from build123d import *

# Parameters (mm, degrees)
F3_DEPTH     = 3.5
F4_SIZE      = 1
F5_SIZE      = 0.5
F6_T4_DEPTH  = 8.4221557451
F6_T11_DEPTH = 13.7150489639
F6_T21_DEPTH = 8.4221557451
F6_T28_DEPTH = 8.4221557451
F6_T35_DEPTH = 13.7150489639
F6_T45_DEPTH = 8.4221557451
F7_R         = 1.5
F8_R         = 1
F9_DEPTH     = 25


# Not quite as in the source:
# - a fillet or chamfer that OpenCascade refuses, or shapes differently, is made with other operations: its cross-section is extruded or revolved along the edge and cut away or added


with BuildPart() as f1:
    # F0 (on Front) → F1 (revolve)
    with BuildSketch(Plane.XZ):
        Polygon((0, 7), (0, 0), (5.5, 0), (5.5, 3.5), (6.5, 3.5), (6.5, 7), align=None)
    revolve(axis=Axis((0, 0, 5.0261294236), (0, 0, 1)))

    # F2 (on Front) → F3 (join, symmetric)
    with BuildSketch(Plane.XZ):
        Polygon((3.5, 0), (-3.5, 0), (-3.5, -2.5), (-2, -2.5), (-2, -7.5), (-3.5, -7.5), (-3.5, -9.5), (3.5, -9.5), (3.5, -7.5), (2, -7.5), (2, -2.5), (3.5, -2.5), align=None)
    extrude(amount=F3_DEPTH, both=True)

    # F4
    f4_edges = [f1.edges().sort_by_distance(p)[0] for p in [
        (3.5, -3.5, -1.25),
        (3.5, 3.5, -1.25),
        (-3.5, 3.5, -1.25),
        (-3.5, -3.5, -1.25),
        (-3.5, -3.5, -8.5),
        (3.5, -3.5, -8.5),
        (-3.5, 3.5, -8.5),
        (3.5, 3.5, -8.5),
    ]]
    chamfer(f4_edges, length=F4_SIZE)

    # F5
    f5_edges = [f1.edges().sort_by_distance(p)[0] for p in [
        (2, -3.5, -5),
        (-2, -3.5, -5),
        (-2, 3.5, -5),
        (2, 3.5, -5),
    ]]
    chamfer(f5_edges, length=F5_SIZE)

    # F6: chamfer of 1.5 on 6 edges, made by hand


with BuildPart() as f6_tool2:
    # F6_s3 → F6_t4 (new body)
    with BuildSketch(Plane(origin=(3.7276817198, -3.7276817198, 0), x_dir=(0, 0, 1), z_dir=(-0.7071067812, 0.7071067812, 0))):
        Polygon((-7.5, -5.0355339059), (-6, -3.5355339059), (-7.5, -3.5355339059), align=None)
    extrude(amount=F6_T4_DEPTH)

    split(bisect_by=Plane.XZ.offset(3.5), keep=Keep.BOTTOM)

    split(bisect_by=Plane(origin=(-3, -3, 0), x_dir=(0, 0, 1), z_dir=(0.7071067812, 0.7071067812, 0)), keep=Keep.TOP)

    split(bisect_by=Plane(origin=(2, 0, -2), x_dir=(0, 1, 0), z_dir=(0.7071067812, 0, -0.7071067812)), keep=Keep.TOP)


with BuildPart() as f1_1:
    add(f1.part)

    # F6_t1: union F6_tool2
    add(f6_tool2.part)


with BuildPart() as f6_tool9:
    # F6_s10 → F6_t11 (new body)
    with BuildSketch(Plane.XZ.offset(-6.8575244819)):
        Polygon((-3.5, -7.5), (-2, -6), (-2, -7.5), align=None)
    extrude(amount=F6_T11_DEPTH)

    split(bisect_by=Plane.XZ.offset(3.5), keep=Keep.BOTTOM)

    split(bisect_by=Plane(origin=(-3, -3, 0), x_dir=(0, 0, 1), z_dir=(0.7071067812, 0.7071067812, 0)), keep=Keep.TOP)

    split(bisect_by=Plane.XZ.offset(-3.5), keep=Keep.TOP)

    split(bisect_by=Plane(origin=(-3, 3, 0), x_dir=(0, 0, 1), z_dir=(0.7071067812, -0.7071067812, 0)), keep=Keep.TOP)

    split(bisect_by=Plane(origin=(0.8713203436, -0.8713203436, -1.232233047), x_dir=(0.7071067812, 0.7071067812, 0), z_dir=(0.5, -0.5, -0.7071067812)), keep=Keep.TOP)

    split(bisect_by=Plane(origin=(0.8713203436, 0.8713203436, -1.232233047), x_dir=(-0.7071067812, 0.7071067812, 0), z_dir=(0.5, 0.5, -0.7071067812)), keep=Keep.TOP)


with BuildPart() as f1_2:
    add(f1_1.part)

    # F6_t8: union F6_tool9
    add(f6_tool9.part)


with BuildPart() as f6_tool19:
    # F6_s20 → F6_t21 (new body)
    with BuildSketch(Plane(origin=(3.7276817198, 3.7276817198, 0), x_dir=(0, 0, 1), z_dir=(-0.7071067812, -0.7071067812, 0))):
        Polygon((-7.5, 5.0355339059), (-6, 3.5355339059), (-7.5, 3.5355339059), align=None)
    extrude(amount=F6_T21_DEPTH)

    split(bisect_by=Plane.XZ.offset(-3.5), keep=Keep.TOP)

    split(bisect_by=Plane(origin=(-3, 3, 0), x_dir=(0, 0, 1), z_dir=(0.7071067812, -0.7071067812, 0)), keep=Keep.TOP)

    split(bisect_by=Plane(origin=(2, 0, -2), x_dir=(0, 1, 0), z_dir=(0.7071067812, 0, -0.7071067812)), keep=Keep.TOP)


with BuildPart() as f1_3:
    add(f1_2.part)

    # F6_t18: union F6_tool19
    add(f6_tool19.part)


with BuildPart() as f6_tool26:
    # F6_s27 → F6_t28 (new body)
    with BuildSketch(Plane(origin=(-3.7276817198, -3.7276817198, 0), x_dir=(0, 0, 1), z_dir=(0.7071067812, 0.7071067812, 0))):
        Polygon((-7.5, 5.0355339059), (-6, 3.5355339059), (-7.5, 3.5355339059), align=None)
    extrude(amount=F6_T28_DEPTH)

    split(bisect_by=Plane.XZ.offset(3.5), keep=Keep.BOTTOM)

    split(bisect_by=Plane(origin=(3, -3, 0), x_dir=(0, 0, 1), z_dir=(-0.7071067812, 0.7071067812, 0)), keep=Keep.TOP)

    split(bisect_by=Plane(origin=(-2, 0, -2), x_dir=(0, 1, 0), z_dir=(-0.7071067812, 0, -0.7071067812)), keep=Keep.TOP)


with BuildPart() as f1_4:
    add(f1_3.part)

    # F6_t25: union F6_tool26
    add(f6_tool26.part)


with BuildPart() as f6_tool33:
    # F6_s34 → F6_t35 (new body)
    with BuildSketch(Plane.XZ.offset(-6.8575244819)):
        Polygon((3.5, -7.5), (2, -6), (2, -7.5), align=None)
    extrude(amount=F6_T35_DEPTH)

    split(bisect_by=Plane.XZ.offset(3.5), keep=Keep.BOTTOM)

    split(bisect_by=Plane(origin=(3, -3, 0), x_dir=(0, 0, 1), z_dir=(-0.7071067812, 0.7071067812, 0)), keep=Keep.TOP)

    split(bisect_by=Plane.XZ.offset(-3.5), keep=Keep.TOP)

    split(bisect_by=Plane(origin=(3, 3, 0), x_dir=(0, 0, 1), z_dir=(-0.7071067812, -0.7071067812, 0)), keep=Keep.TOP)

    split(bisect_by=Plane(origin=(-0.8713203436, -0.8713203436, -1.232233047), x_dir=(0.7071067812, -0.7071067812, 0), z_dir=(-0.5, -0.5, -0.7071067812)), keep=Keep.TOP)

    split(bisect_by=Plane(origin=(-0.8713203436, 0.8713203436, -1.232233047), x_dir=(-0.7071067812, -0.7071067812, 0), z_dir=(-0.5, 0.5, -0.7071067812)), keep=Keep.TOP)


with BuildPart() as f1_5:
    add(f1_4.part)

    # F6_t32: union F6_tool33
    add(f6_tool33.part)


with BuildPart() as f6_tool43:
    # F6_s44 → F6_t45 (new body)
    with BuildSketch(Plane(origin=(-3.7276817198, 3.7276817198, 0), x_dir=(0, 0, 1), z_dir=(0.7071067812, -0.7071067812, 0))):
        Polygon((-7.5, -5.0355339059), (-6, -3.5355339059), (-7.5, -3.5355339059), align=None)
    extrude(amount=F6_T45_DEPTH)

    split(bisect_by=Plane.XZ.offset(-3.5), keep=Keep.TOP)

    split(bisect_by=Plane(origin=(3, 3, 0), x_dir=(0, 0, 1), z_dir=(-0.7071067812, -0.7071067812, 0)), keep=Keep.TOP)

    split(bisect_by=Plane(origin=(-2, 0, -2), x_dir=(0, 1, 0), z_dir=(-0.7071067812, 0, -0.7071067812)), keep=Keep.TOP)


with BuildPart() as f1_6:
    add(f1_5.part)

    # F6_t42: union F6_tool43
    add(f6_tool43.part)

    # F7
    f7_edges = [f1_6.edges().sort_by_distance(p)[0] for p in [
        (-6.5, 0, 7),
    ]]
    fillet(f7_edges, radius=F7_R)

    # F8 (on face) → F9 (cut)
    with BuildSketch(Plane(origin=(0, 0, -9.5), x_dir=(1, 0, 0), z_dir=(0, 0, -1))):
        Circle(F8_R)
    extrude(amount=-F9_DEPTH, mode=Mode.SUBTRACT)


solid = f1_6.part
CAD build for the part. Positions are in the model's coordinates, mm. A direction names the side the tool comes from. Round coordinates to 2 decimals unless told otherwise and drop trailing zeros. Write each loop counter-clockwise with the first axis right and the second up, starting at its lowest first coordinate (ties: lowest second). Pieces come first, ordered by that corner, then holes. Notation, with made-up numbers: M 41.5,-0.5 L 72.5,-0.5 A24 ccw 72.5,26.5 Z; hole C -11,29 d8. An arc over 180 degrees is marked long. Use a Markdown table: item, result. Add a question column.
1. 3-axis set-ups, long thin cutter, end or side, ignore diameter. For faces 5 (the face through (-3.5, 0, -8)), 6 (the face through (0, -3.5, -5)), 7 (the face through (-3, -3, -1)), 8 (the face through (-3, 3, -1)): which of +Z, -Z, +X, -X, +Y, -Y reach the whole face in a straight line?
2. Slice it at B-B on x = 0. Give the cut face in (y, z), then the cut area to 3 significant figures.
3. Slice it at D-D on z = 4.25. Give the cut face in (x, y), then the cut area to 3 significant figures.
4. Drill centre lines: probe 1 along Y at (x, z) = (0, -5.25); probe 2 along Y at (x, z) = (0, 1). Where is each one in solid material? Low to high.
5. Pull direction Z, two halves, no side cores. Call faces 1 (the face through (3, 0, -2.5)), 2 (the face through (3.5, 0, -1)), 3 (the face through (2, 0, -4)), 4 (the face through (-1, -1, -9.5)): released by +Z, released by -Z, zero draft, split by the parting line, or undercut.
6. Flat gauge pins, fed straight in: P1, Ø4, axis at x = -2, z = -7.5, coming from the -Y side; P2, Ø0.8, axis at y = 1, z = -1.5, coming from the -X side; P3, Ø1.5, axis at x = -3.5, z = -2, coming from the -Y side. Where does each tip first touch, or does it go through?
7. Slice it at C-C on z = -1.5. Give the cut face in (x, y), then the cut area to 3 significant figures.
8. Slice it at A-A on y = 0. Give the cut face in (x, z), then the cut area to 3 significant figures.
Reply:
| question | item | result |
|---|---|---|
| 1 | face 5 | -Z, -X, +Y, -Y |
| 1 | face 6 | -Z, +X, -X, -Y |
| 1 | face 7 | -Z, -X, -Y |
| 1 | face 8 | -Z, -X, +Y |
| 2 | outline | M -6.5,3.5 L -5.5,3.5 L -5.5,0 L -3.5,0 L -3.5,-9.5 L -1,-9.5 L -1,7 L -5,7 A1.5 ccw -6.5,5.5 Z; M 1,-9.5 L 3.5,-9.5 L 3.5,0 L 5.5,0 L 5.5,3.5 L 6.5,3.5 L 6.5,5.5 A1.5 ccw 5,7 L 1,7 Z |
| 2 | area | 117 mm^2 |
| 3 | outline | C 0,0 d13; hole C 0,0 d2 |
| 3 | area | 130 mm^2 |
| 4 | probe 1 | y = -3.5 to -1, 1 to 3.5 |
| 4 | probe 2 | y = -5.5 to -1, 1 to 5.5 |
| 5 | face 1 | undercut |
| 5 | face 2 | zero draft |
| 5 | face 3 | undercut |
| 5 | face 4 | released by -Z |
| 6 | P1 | stops at y = -3.5 |
| 6 | P2 | stops at x = -3.5 |
| 6 | P3 | stops at y = -3.25 |
| 7 | outline | M -3.5,-2.5 L -2.5,-3.5 L 2.5,-3.5 L 3.5,-2.5 L 3.5,2.5 L 2.5,3.5 L -2.5,3.5 L -3.5,2.5 Z; hole C 0,0 d2 |
| 7 | area | 43.9 mm^2 |
| 8 | outline | M -6.5,3.5 L -5.5,3.5 L -5.5,0 L -3.5,0 L -3.5,-2.5 L -2,-2.5 L -2,-6 L -3.5,-7.5 L -3.5,-9.5 L -1,-9.5 L -1,7 L -5,7 A1.5 ccw -6.5,5.5 Z; M 1,-9.5 L 3.5,-9.5 L 3.5,-7.5 L 2,-6 L 2,-2.5 L 3.5,-2.5 L 3.5,0 L 5.5,0 L 5.5,3.5 L 6.5,3.5 L 6.5,5.5 A1.5 ccw 5,7 L 1,7 Z |
| 8 | area | 104 mm^2 |
